Model file for the job. Use its own axes, mm. A direction names the side the tool comes from. Give positions to 0.01 mm unless a question says otherwise; leave off trailing zeros. Write each loop counter-clockwise with the first axis right and the second up, starting at its lowest first coordinate (ties: lowest second). Pieces come first, ordered by that corner, then holes. Notation, with made-up numbers: M 62,31.25 L 80,31.25 A20 ccw 80,58.25 Z; hole C 70.25,-10 d2. An arc over 180 degrees is marked long. Answer as a JSON object with one key per item and string values. Group by question number.
```python
from build123d import *

# Parameters (mm, degrees)
BOSS_EXTRUDE1_DEPTH     = 15.875
SKETCH4_R               = 3.175
CUT_EXTRUDE1_DEPTH      = 49.464271634
SKETCH3_OUTSIDE_W       = 54.3
SKETCH3_OUTSIDE_H       = 47.95
CUT_EXTRUDE2_DEPTH      = 57.529267862
F_1_4_CLEARANCE_HOLE1_D = 6.5278
SKETCH9_R               = 6.35
CUT_EXTRUDE3_DEPTH      = 2.54


with BuildPart() as part:
    # Sketch2 → Boss-Extrude1 (new, symmetric)
    with BuildSketch(Plane.XY):
        with BuildLine():
            Line((-19.05, -25.4), (19.05, -25.4))
            Line((19.05, -25.4), (19.05, 25.4))
            Line((19.05, 25.4), (17.4625, 25.4))
            ThreePointArc((17.4625, 25.4), (16.339967985, 24.935032015), (15.875, 23.8125))
            Line((15.875, 23.8125), (15.875, -17.4498))
            ThreePointArc((15.875, -17.4498), (14.476376302, -20.826376302), (11.0998, -22.225))
            Line((11.0998, -22.225), (-17.4625, -22.225))
            ThreePointArc((-17.4625, -22.225), (-18.585032015, -22.689967985), (-19.05, -23.8125))
            Line((-19.05, -23.8125), (-19.05, -25.4))
        make_face()
    extrude(amount=BOSS_EXTRUDE1_DEPTH, both=True)

    # Sketch4 → Cut-Extrude1 (cut, through all)
    with BuildSketch(Plane(origin=(19.05, 0, 0), x_dir=(0, 0, -1), z_dir=(1, 0, 0))):
        with Locations(Location((-3.175, 12.7, 0), (0, 0, 90))):
            Circle(SKETCH4_R)
        with Locations(Location((-3.175, -12.7, 0), (0, 0, 90))):
            Circle(SKETCH4_R)
    extrude(amount=-CUT_EXTRUDE1_DEPTH, mode=Mode.SUBTRACT)

    # Sketch3 outside → Cut-Extrude2 (cut, through all)
    with BuildSketch(Plane.XZ.offset(25.4)):
        Rectangle(SKETCH3_OUTSIDE_W, SKETCH3_OUTSIDE_H)
        Polygon((-19.05, 13.926834826), (-19.05, -11.481872103), (19.05, -10.484188491), (19.05, 14.924518438), align=None, mode=Mode.SUBTRACT)
    extrude(amount=-CUT_EXTRUDE2_DEPTH, mode=Mode.SUBTRACT)

    # 1/4 Clearance Hole1 (through all)
    with Locations(Plane(origin=(0, -25.4, 0), x_dir=(-1, 0, 0), z_dir=(0, -1, 0))):
        with Locations((6.021904729, -1.56363455)):
            Hole(F_1_4_CLEARANCE_HOLE1_D / 2)

    # Sketch9 → Cut-Extrude3 (cut)
    with BuildSketch(Plane.ZY.offset(-15.875)):
        with Locations((3.175, -12.7)):
            Circle(SKETCH9_R)
    extrude(amount=CUT_EXTRUDE3_DEPTH, mode=Mode.SUBTRACT)


solid = part.part
```
Q1. Slice it at D-D, the plane y = 2. Write the cut outline in (x, z) (3 decimals), then the cut area to 3 significant figures.
Q2. Wall check: L1, parallel to Z at x = 16.9, y = -12.7; L2, parallel to Y at x = -10.5, z = 9.75 (3 decimals); L3, parallel to X at y = -17.5, z = -6.25. Give the ranges that are in metal, low to high.
Q3. 3-axis set-ups, long thin cutter, end or side, ignore diameter. For faces 3 (the flat face through (0, -25.4, 2)), 4 (the flat face through (-3, -22.225, 5)): which of +Z, -Z, +X, -X, +Y, -Y reach the whole face in a straight line?
Q4. Two-plate mould, pull along Z, no slides. Class faces 1 (the flat face through (-19.05, -25, 1)), 2 (the cylindrical face through (17.48, -9.67, 4.13)): +Z half, -Z half, draft (parallel to the pull), parting line (faces both ways), or undercut.
Q5. Slice it at C-C, the plane x = -6. Write the cut outline in (y, z) (3 decimals).
Q6. Slice it at A-A, the plane y = -12.7. Write the cut outline in (x, z) (3 decimals).
Q7. Drop flat-ended pins along their axis: P1, Ø1.5, axis at x = 14, z = 2.5, coming from the +Y side; P2, Ø12, axis at y = 1, z = 2, coming from the -X side (3 decimals); P3, Ø3, axis at x = 1, z = 8, coming from the +Y side (3 decimals). Give the stop position or say it passes through.
Solved:
{
 "1": {"outline": "M 15.875,-10.567 L 19.05,-10.484 L 19.05,14.925 L 15.875,14.841 Z", "area": "80.7 mm²"},
 "2": {"L1": "z = -10.54 to 0, 6.35 to 14.87", "L2": "y = -25.4 to -22.225", "L3": "x = 15.87 to 19.05"},
 "3": {"face 3": "+Z, -Z, +X, -X, -Y", "face 4": "+Z, -Z, -X, +Y"},
 "4": {"face 1": "draft", "face 2": "undercut"},
 "5": {"outline": "M -25.4,-11.14 L -22.225,-11.14 L -22.225,-1.7 L -25.4,-1.7 Z; M -25.4,4.827 L -22.225,4.827 L -22.225,14.269 L -25.4,14.269 Z"},
 "6": {"outline": "M 15.875,-10.567 L 19.05,-10.484 L 19.05,0 L 15.875,0 Z; M 15.875,6.35 L 19.05,6.35 L 19.05,14.925 L 15.875,14.841 Z"},
 "7": {"P1": "stops at y = -20.53", "P2": "stops at x = 15.875", "P3": "stops at y = -22.225"}
}
